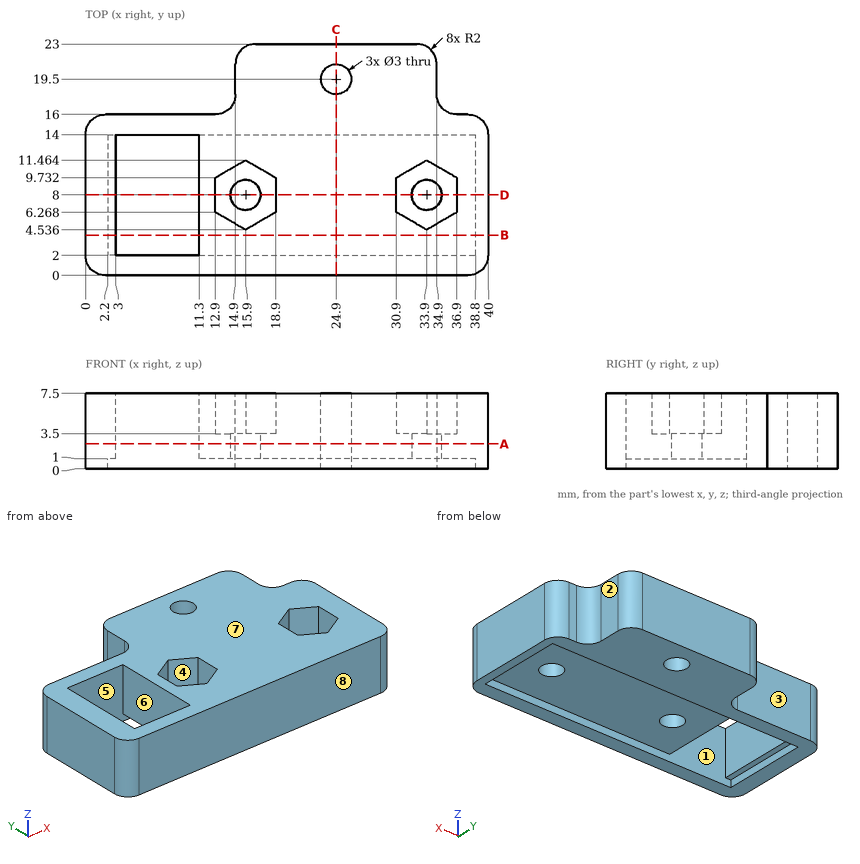
Study the drawing (mm; zero at the part's minimum x, y, z) and answer. A direction names the side the tool comes from. Give positions to 0.01 mm unless a question says otherwise; leave off trailing zeros. Order: outer loops, then holes, each group sorted by start corner. A loop starts at its lowest first (then second) coordinate and runs counter-clockwise, first axis right, second up. Notation, with made-up numbers: (-7, -24) -> (3, -24) arc R13 cw to (3, -6) -> close; hole circle Ø10 at (-27, 21.25). An arc over 180 degrees is marked (long way). Put each result on its own line as item: value.
Item 1: A cutting plane is placed at D-D on y = 8. Give the vertices of the cut face in (x, z).
Established:
outline: (0, 0) -> (2.2, 0) -> (2.2, 1) -> (3, 1) -> (3, 7.5) -> (0, 7.5) -> close; (11.3, 1) -> (14.4, 1) -> (14.4, 3.5) -> (12.9, 3.5) -> (12.9, 7.5) -> (11.3, 7.5) -> close; (17.4, 1) -> (32.4, 1) -> (32.4, 3.5) -> (30.9, 3.5) -> (30.9, 7.5) -> (18.9, 7.5) -> (18.9, 3.5) -> (17.4, 3.5) -> close; (35.4, 1) -> (38.8, 1) -> (38.8, 0) -> (40, 0) -> (40, 7.5) -> (36.9, 7.5) -> (36.9, 3.5) -> (35.4, 3.5) -> close
Item 2: A cutting plane is placed at A-A on z = 2.5. Give the vertices of the cut face in (x, y).
Established:
outline: (0, 2) arc R2 ccw to (2, 0) -> (38, 0) arc R2 ccw to (40, 2) -> (40, 14) arc R2 ccw to (38, 16) -> (36.9, 16) arc R2 cw to (34.9, 18) -> (34.9, 21) arc R2 ccw to (32.9, 23) -> (16.9, 23) arc R2 ccw to (14.9, 21) -> (14.9, 18) arc R2 cw to (12.9, 16) -> (2, 16) arc R2 ccw to (0, 14) -> close; hole (3, 2) -> (11.3, 2) -> (11.3, 14) -> (3, 14) -> close; hole circle Ø3 at (15.9, 8); hole circle Ø3 at (24.9, 19.5); hole circle Ø3 at (33.9, 8)
Item 3: For a pull along Y with two mould halves and no side action, classify the marked faces 5, 6, 7 and 8 as released by +Y, released by -Y, zero draft, split by the parting line, or undercut.
Established:
face 5: undercut
face 6: undercut
face 7: zero draft
face 8: released by -Y
Item 4: Straight lines are drawn through the part: line 1 (X direction, y = 8, z = 2.6); line 2 (Y direction, x = 2, z = 3.75); line 3 (X direction, y = 12, z = 4). For each, find the intervals that lie inside material, in ascending order.
Established:
line 1: x = 0 to 3, 11.3 to 14.4, 17.4 to 32.4, 35.4 to 40
line 2: y = 0 to 16
line 3: x = 0 to 3, 11.3 to 40
Item 5: For the marked faces 1, 2, 3 and 4, determine the directions among +Z, -Z, +X, -X, +Y, -Y from which every point of the face is accessible in a straight line to the end or side of a thin tool.
Established:
face 1: -Z
face 2: +Z, -Z, +X, +Y
face 3: +Z, -Z, -X, +Y
face 4: +Z
Item 6: Given P1, Ø3, axis at x = 16.5, y = 7, coming from the +Z side; P2, Ø4, axis at x = 15.9, y = 8, coming from the -Z side; P3, Ø2, axis at x = 5.5, z = 3.5, coming from the +Y side; P4, Ø1.8, axis at x = 33.9, y = 8, coming from the -Z side, each flat-ended and moving along its own axis, determine where each tip first touches the part or whether it passes through.
Established:
P1: stops at z = 3.5
P2: stops at z = 1
P3: stops at y = 16
P4: passes through
Item 7: A cutting plane is placed at C-C on x = 24.9. Give the vertices of the cut face in (y, z), plus the area to 3 significant figures.
Established:
outline: (0, 0) -> (2, 0) -> (2, 1) -> (14, 1) -> (14, 0) -> (18, 0) -> (18, 7.5) -> (0, 7.5) -> close; (21, 0) -> (23, 0) -> (23, 7.5) -> (21, 7.5) -> close
area: 138 mm^2
Item 8: A cutting plane is placed at B-B on y = 4. Give the vertices of the cut face in (x, z), plus the area to 3 significant figures.
Established:
outline: (0, 0) -> (2.2, 0) -> (2.2, 1) -> (3, 1) -> (3, 7.5) -> (0, 7.5) -> close; (11.3, 1) -> (38.8, 1) -> (38.8, 0) -> (40, 0) -> (40, 7.5) -> (11.3, 7.5) -> close
area: 209 mm^2
